Input: part model. Units: mm. Frame: model coordinates. A direction names the side the tool comes from. Round coordinates to 2 decimals unless told otherwise and drop trailing zeros. Write each loop counter-clockwise with the first axis right and the second up, starting at its lowest first coordinate (ties: lowest second). Pieces come first, ordered by that corner, then holes. Notation, with made-up numbers: (57, -14.5) -> (69, -14.5) arc R16 cw to (69, 6.5) -> close; hole circle Ø6 at (15.25, 43.5). An arc over 180 degrees is marked (long way). Use CSV: the item, a comma, the result in double quotes.
```python
from build123d import *

# Parameters (mm, degrees)
SKETCH1_W           = 70
SKETCH1_H           = 70
BOSS_EXTRUDE1_DEPTH = 250
SKETCH2_R           = 30
CUT_EXTRUDE2_DEPTH  = 65
SKETCH4_R           = 5
CUT_EXTRUDE3_DEPTH  = 261.672207955


with BuildPart() as part:
    # Sketch1 → Boss-Extrude1 (new body)
    with BuildSketch(Plane(origin=(0, 0, 0), x_dir=(1, 0, 0), z_dir=(0, 1, 0))):
        Rectangle(SKETCH1_W, SKETCH1_H)
    extrude(amount=BOSS_EXTRUDE1_DEPTH)

    # Sketch2 → Cut-Extrude2 (cut)
    with BuildSketch(Plane.XY.offset(35)):
        with BuildLine():
            Line((-35, 250), (-35, 215))
            ThreePointArc((-35, 215), (-24.748737311, 239.748737372), (8.5e-08, 250))
            Line((8.5e-08, 250), (-35, 250))
        make_face()
        with BuildLine():
            Line((35, 250), (8.5e-08, 250))
            ThreePointArc((8.5e-08, 250), (24.748737372, 239.748737311), (35, 215))
            Line((35, 215), (35, 250))
        make_face()
        with BuildLine():
            ThreePointArc((1.6e-08, 0), (-24.748737336, 10.251262653), (-35, 35))
            Line((-35, 35), (-35, 0))
            Line((-35, 0), (1.6e-08, 0))
        make_face()
        with BuildLine():
            ThreePointArc((35, 35), (24.748737347, 10.251262664), (1.6e-08, 0))
            Line((1.6e-08, 0), (35, 0))
            Line((35, 0), (35, 35))
        make_face()
        with BuildLine():
            ThreePointArc((30, 215), (0, 185), (-30, 215))
            Line((-30, 215), (-30, 35))
            ThreePointArc((-30, 35), (0, 65), (30, 35))
            Line((30, 35), (30, 215))
        make_face()
        with Locations((0, 215)):
            Circle(SKETCH2_R)
        with Locations((0, 35)):
            Circle(SKETCH2_R)
    extrude(amount=-CUT_EXTRUDE2_DEPTH, mode=Mode.SUBTRACT)

    # Sketch4 → Cut-Extrude3 (cut, through all)
    with BuildSketch(Plane.XY.offset(-30)):
        with BuildLine():
            ThreePointArc((1.9e-08, 0), (-24.748737335, 10.251262652), (-35, 35))
            Line((-35, 35), (-35, 0))
            Line((-35, 0), (1.9e-08, 0))
        make_face()
        with BuildLine():
            Line((35, 0), (35, 35))
            ThreePointArc((35, 35), (24.748737348, 10.251262665), (1.9e-08, 0))
            Line((1.9e-08, 0), (35, 0))
        make_face()
        with BuildLine():
            Line((-35, 250), (-35, 215))
            ThreePointArc((-35, 215), (-24.748737474, 239.748737209), (-3.75e-07, 250))
            Line((-3.75e-07, 250), (-35, 250))
        make_face()
        with BuildLine():
            ThreePointArc((-3.75e-07, 250), (24.748737209, 239.748737474), (35, 215))
            Line((35, 215), (35, 250))
            Line((35, 250), (-3.75e-07, 250))
        make_face()
        with Locations((0, 215)):
            Circle(SKETCH4_R)
        with Locations((0, 35)):
            Circle(SKETCH4_R)
    extrude(amount=-CUT_EXTRUDE3_DEPTH, mode=Mode.SUBTRACT)


solid = part.part
```
Item 1: Section query A-A on y = 108. Return the cut outline in (x, z), plus the area to 3 significant figures.
Worked answers:
outline,"(-35, -35) -> (35, -35) -> (35, 35) -> (30, 35) -> (30, -30) -> (-30, -30) -> (-30, 35) -> (-35, 35) -> close"
area,"1,000 mm²"
Item 2: First-contact query: pin 1 Ø3 at (x, z) = (17.5, -16.5) entering from -Y; pin 2 Ø12 at (x, z) = (-28, 26.5) entering from +Y; pin 3 Ø4 at (x, z) = (-20, 16) entering from +Y. Flat tips, straight axial feed; report the tip coordinate or a pass-through.
Worked answers:
pin 1,"stops at y = 3.87"
pin 2,"stops at y = 242.22"
pin 3,"stops at y = 245.02"
Item 3: Section query B-B on z = -7. Return the cut outline in (x, y).
Worked answers:
outline,"(-35, 35) arc R35 ccw to (35, 35) -> (35, 215) arc R35 ccw to (-35, 215) -> close; hole (-30, 35) arc R30 ccw to (30, 35) -> (30, 215) arc R30 ccw to (-30, 215) -> close"
Item 4: Set-up query: faces 1 (the face through (-0.651, 219.957, -32.465)), 2 (the face through (0, 127, -30)). Return all of +Z, -Z, +X, -X, +Y, -Y with unobstructed straight access to the full face (end or side cutting, diameter ignored); none if empty.
Worked answers:
face 1,"+Z, -Z"
face 2,"+Z"
Item 5: Line query: line 1 (X direction, y = 202.5, z = 29.5); line 2 (Z direction, x = 25, y = 53); line 3 (Y direction, x = -12, z = -26.5). Output: solid intervals per line, ascending.
Worked answers:
line 1,"x = -35 to -30, 30 to 35"
line 2,"z = -35 to -30"
line 3,"y = 2.12 to 7.5, 242.5 to 247.88"
Item 6: Section query C-C on x = 7.5. Return the cut outline in (y, z).
Worked answers:
outline,"(0.81, -35) -> (249.19, -35) -> (249.19, 35) -> (244.05, 35) -> (244.05, -30) -> (5.95, -30) -> (5.95, 35) -> (0.81, 35) -> close"
Item 7: Pull-direction query (Y, two-part tool) for faces 3 (the face through (0.77, 0.01, 0.49)), 4 (the face through (-35, 124, 0)), 5 (the face through (30, 124, 3)); classes: +Y half, -Y half, draft (parallel to the pull), parting line (faces both ways), or undercut.
Worked answers:
face 3,"-Y half"
face 4,"draft"
face 5,"undercut"
